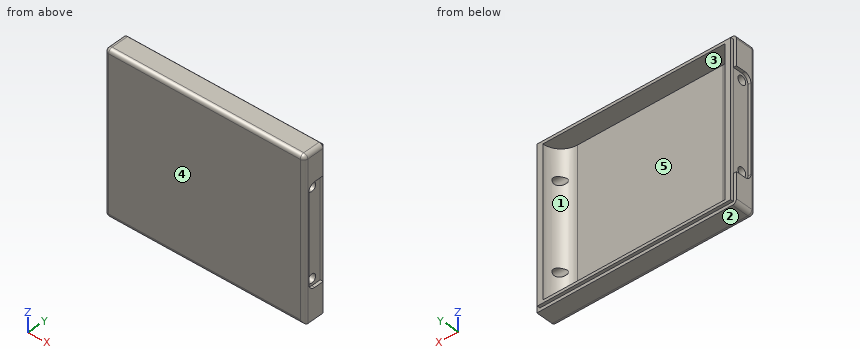
Autodesk Inventor part; units mm, degrees
ref_plane "YZ Plane" through (0, 0, 0) normal (1, 0, 0) x (0, 1, 0)
ref_plane "XZ Plane" through (0, 0, 0) normal (0, 1, 0) x (-1, 0, 0)
ref_plane "XY Plane" through (0, 0, 0) normal (0, 0, 1) x (1, 0, 0)
sketch "草圖1" plane through (0, 0, 0) normal (0, 1, 0) x (-1, 0, 0)
  line L0 (50, 40) -> (-50, 40)
  line L1 (-50, 40) -> (-50, -40)
  line L2 (-50, -40) -> (50, -40)
  line L3 (50, -40) -> (50, 40)
  line L4 (50, 40) -> (-50, -40) construction
  line L5 (-50, 40) -> (50, -40) construction
  point P0 (0, 0)
  dimension "d0" = 100
  dimension "d1" = 80
extrude "擠出1" add sketch "草圖1" along normal blind 3
sketch "草圖2" plane through (0, 3, 0) normal (0, 1, 0) x (1, 0, 0)
  line L0 (50, -40) -> (50, 40)
  line L1 (50, 40) -> (-50, 40)
  line L2 (-50, 40) -> (-50, -40)
  line L3 (-50, -40) -> (50, -40)
  line L4 (-47, -37) -> (-47, 37)
  line L5 (-47, 37) -> (47, 37)
  line L6 (47, 37) -> (47, -37)
  line L7 (47, -37) -> (-47, -37)
  point P0 (0, 0)
  dimension "d4" = 3
extrude "擠出2" add sketch "草圖2" along normal blind 9.125
sketch "草圖3" plane through (-47, 3, -37) normal (0, 0, 1) x (1, 0, 0)
  line L0 (94, 0) -> (0, 0)
  line L1 (94, 0) -> (94, 9.125)
  line L2 (0, 9.125) -> (94, 9.125)
  line L3 (0, 0) -> (0, 9.125)
  circle A0 centre (10.5, 9.125) radius 9.125
  circle A1 centre (28.75, 9.125) radius 9.125
  circle A2 centre (47, 9.125) radius 9.125
  circle A3 centre (65.25, 9.125) radius 9.125
  circle A4 centre (83.5, 9.125) radius 9.125
  point P0 (47, -3)
  point P1 (92.625, 9.125)
  point P2 (83.5, 0)
  point P3 (10.5, 0)
  point P4 (1.375, 9.125)
  dimension "d7" = 18.25
  dimension "d11" = 18.25
  dimension "d16" = 10.5
extrude "擠出3" add sketch "草圖3" along normal through all contours L0 A4 L2 L1 | L0 L3 L2 A0
sketch "草圖4" plane through (0, 12.125, 0) normal (0, 1, 0) x (1, 0, 0)
  line L0 (-50, -40) -> (50, -40)
  line L1 (50, -40) -> (50, 40)
  line L2 (50, 40) -> (-50, 40)
  line L3 (-50, 40) -> (-50, -40)
  line L4 (45.625, -37) -> (-45.625, -37)
  line L5 (-45.625, 37) -> (-45.625, -37)
  line L6 (-45.625, 37) -> (45.625, 37)
  line L7 (45.625, 37) -> (45.625, -37)
  line L8 (48.5, -38.5) -> (-48.5, -38.5)
  line L9 (-48.5, -38.5) -> (-48.5, 38.5)
  line L10 (-48.5, 38.5) -> (48.5, 38.5)
  line L11 (48.5, 38.5) -> (48.5, -38.5)
  line L12 (-48.45, -38.45) -> (48.45, -38.45)
  line L13 (48.45, -38.45) -> (48.45, 38.45)
  line L14 (48.45, 38.45) -> (-48.45, 38.45)
  line L15 (-48.45, 38.45) -> (-48.45, -38.45)
  point P0 (0, 0)
  dimension "d19" = 1.5
  dimension "d20" = 0.05
extrude "擠出4" cut sketch "草圖4" against normal blind 1.51 contours L3 L2 L1 L0 | L8 L9 L10 L11
sketch "草圖5" plane through (50, 0, 40) normal (1, 0, 0) x (0, 0, -1)
  circle A0 centre (18.3, 5.925) radius 1.65
  circle A1 centre (61.7, 5.925) radius 1.65
  line L0 (28.79, 21.325) -> (15, 21.325)
  line L1 (15, 21.325) -> (15, 27.625)
  line L2 (15, 27.625) -> (28.79, 27.625)
  line L3 (28.79, 27.625) -> (28.79, 21.325)
  line L4 (51.21, 21.325) -> (51.21, 27.625)
  line L5 (51.21, 27.625) -> (65, 27.625)
  line L6 (65, 27.625) -> (65, 21.325)
  line L7 (65, 21.325) -> (51.21, 21.325)
  line L8 (15, 10.625) -> (2, 10.625)
  line L9 (15, 10.625) -> (15, 5.925)
  arc A2 (15, 5.925) -> (18.3, 2.625) centre (18.3, 5.925) ccw
  line L10 (18.3, 2.625) -> (61.7, 2.625)
  arc A3 (61.7, 2.625) -> (65, 5.925) centre (61.7, 5.925) ccw
  line L11 (65, 5.925) -> (65, 10.625)
  line L12 (78, 10.625) -> (65, 10.625)
  line L13 (15, 10.625) -> (65, 10.625)
  line L14 (80, 10.615) -> (0, 10.615)
  arc A4 (14.9, 5.925) -> (18.3, 2.525) centre (18.3, 5.925) ccw
  line L15 (14.9, 5.925) -> (14.9, 10.525)
  line L16 (14.9, 10.525) -> (-0.1, 10.525)
  line L17 (-0.1, 10.525) -> (-0.1, 30.725)
  line L18 (-0.1, 30.725) -> (80.1, 30.725)
  line L19 (80.1, 30.725) -> (80.1, 10.525)
  line L20 (80.1, 10.525) -> (65.1, 10.525)
  line L21 (65.1, 10.525) -> (65.1, 5.925)
  arc A5 (61.7, 2.525) -> (65.1, 5.925) centre (61.7, 5.925) ccw
  line L22 (61.7, 2.525) -> (18.3, 2.525)
  line L23 (14.9, 10.525) -> (14.9, 10.615)
  line L24 (65.1, 10.525) -> (65.1, 10.615)
  line L25 (78, 28.625) -> (78, 10.625)
  line L26 (2, 10.625) -> (2, 28.625)
  line L27 (46.57, 28.625) -> (46.57, 21.325)
  line L28 (46.57, 21.325) -> (33.43, 21.325)
  line L29 (33.43, 21.325) -> (33.43, 28.625)
  line L30 (46.57, 28.625) -> (78, 28.625)
  line L31 (2, 28.625) -> (33.43, 28.625)
  point P0 (40, 0)
  dimension "d23" = 0.1
extrude "擠出5" cut sketch "草圖5" against normal blind 1.51 contours A0 | A1 | L14 L11 A3 L10 A2 L9 | L9 A2 L10 A3 L11 L14 L24 L21 A5 L22 A4 L15 L23
mirror "鏡射1" about plane through (0, 0, 0) normal (1, 0, 0) of "擠出5"
sketch "草圖6" plane through (48.49, 0, 40) normal (1, 0, 0) x (0, 0, -1)
  circle A0 centre (18.3, 5.925) radius 1.65
  circle A1 centre (61.7, 5.925) radius 1.65
  circle A2 centre (18.3, 5.925) radius 2.165
  circle A3 centre (61.7, 5.925) radius 2.165
  point P0 (40, 0)
  dimension "d26" = 4.33
  dimension "d27" = 4.33
extrude "擠出6" cut sketch "草圖6" against normal through all contours A0 | A1 | A2 | A3
fillet "圓角1" radius 2 7 edges at (-50, 5.3075, 40) (0, 0, 40) (50, 5.3075, 40) (50, 0, 0) (0, 0, -40) (-50, 0, 0) (-50, 5.3075, -40)
properties part number "buttom case_3D 列印"
Design review of the part built by this model. Coordinates are the model's own, in mm. Face numbers are marked on the shaded views. A direction names the side the tool comes from. Coordinates: 2 decimals unless noted, no trailing zeros. Write each loop counter-clockwise with the first axis right and the second up, starting at its lowest first coordinate (ties: lowest second). Pieces come first, ordered by that corner, then holes. Notation, with made-up numbers: (32, 89.25) - (46, 89.25) arc R31 cw to (46, 114.25) - close; hole circle Ø7 at (70.5, -31.75). An arc over 180 degrees is marked (long way). Use one line per item in the form item = value.
Q1. The part is to be moulded in two halves that separate along X. For the marked faces 1, 2 and 3, say which applies: +X half, -X half, draft (parallel to the pull), parting line (faces both ways), or undercut.
Taken from the geometry:
face_1 = undercut
face_2 = draft
face_3 = undercut
Q2. Consider section A-A (z = 27). Write out the cut boundary in (x, y) (3 decimals).
Taken from the geometry:
outline = (-50, 2) arc R2 ccw to (-48, 0) - (48, 0) arc R2 ccw to (50, 2) - (50, 10.615) - (48.45, 10.615) - (48.45, 12.125) - (45.625, 12.125) arc R9.125 cw to (36.5, 3) - (-36.5, 3) arc R9.125 cw to (-45.625, 12.125) - (-48.45, 12.125) - (-48.45, 10.615) - (-50, 10.615) - close
Q3. Insertion check: pin 1 Ø1.2 at (y, z) = (11.5, -15) entering from -X; pin 2 Ø8 at (x, z) = (36.5, -21) entering from +Y; pin 3 Ø5.5 at (y, z) = (5.925, 21.7) entering from +X. Each pin has a flat end and moves straight along its axis. Give the tip position at first contact, or say it passes through.
Taken from the geometry:
pin_1 = -48.45
pin_2 = 3.92
pin_3 = 48.49
Q4. For probe 1 along Z at (x, y) = (-28.5, 6.75); probe 2 along Z at (x, y) = (42.5, 4.5); probe 3 along Y at (x, z) = (45.75, 21.7) (3 decimals), list the stretches that pass through material, from the lowest coordinate up.
Taken from the geometry:
probe_1 = -40 to -37, 37 to 40
probe_2 = -40 to -23.33, -20.07 to 20.07, 23.33 to 40
probe_3 = 0 to 3.76, 8.09 to 12.125
Q5. Consider section B-B (z = -4). Write out the cut boundary in (x, y) (3 decimals), plus the area to 3 significant figures.
Taken from the geometry:
outline = (-50, 2) arc R2 ccw to (-48, 0) - (48, 0) arc R2 ccw to (50, 2) - (50, 2.525) - (48.49, 2.525) - (48.49, 10.615) - (48.45, 10.615) - (48.45, 12.125) - (45.625, 12.125) arc R9.125 cw to (36.5, 3) - (-36.5, 3) arc R9.125 cw to (-45.625, 12.125) - (-48.45, 12.125) - (-48.45, 10.615) - (-48.49, 10.615) - (-48.49, 2.525) - (-50, 2.525) - close
area = 385 mm^2
Q6. Machinability: for the marked faces 4 and 5, which of the approach directions +Z, -Z, +X, -X, +Y, -Y give a long, thin tool a straight path to every point of the face, cutting with its end or side? Answer none if there is none.
Taken from the geometry:
face_4 = +Z, -Z, +X, -X, -Y
face_5 = +Y
